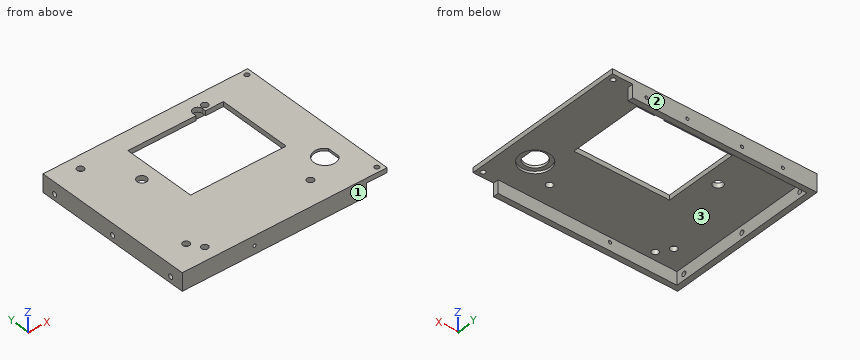
from build123d import *

# Parameters (mm, degrees)
COPYSKETCH010_W   = 150
COPYSKETCH010_H   = 120
COPYSKETCH010_R   = 2.5
COPYSKETCH010_R_2 = 3.5
COPYSKETCH010_R_3 = 1.75
PAD_DEPTH         = 3.5
PAD001_DEPTH      = 13
SKETCH001_R       = 1.75
POCKET_DEPTH      = 5
SKETCH002_R       = 1.15
POCKET001_DEPTH   = 5
SKETCH003_R       = 1.15
POCKET002_DEPTH   = 5
SKETCH004_R       = 11
POCKET003_DEPTH   = 1.75


with BuildPart() as part:
    # CopySketch010 → Pad (new body)
    with BuildSketch(Plane(origin=(0, 0, 0), x_dir=(-1, 0, 0), z_dir=(0, 0, -1))):
        with Locations((-75, 0)):
            Rectangle(COPYSKETCH010_W, COPYSKETCH010_H)
        with Locations((-110, 50)):
            Circle(COPYSKETCH010_R, mode=Mode.SUBTRACT)
        with Locations((-110, -41)):
            Circle(COPYSKETCH010_R, mode=Mode.SUBTRACT)
        with Locations((-19, -41)):
            Circle(COPYSKETCH010_R, mode=Mode.SUBTRACT)
        with Locations((-19, 50)):
            Circle(COPYSKETCH010_R, mode=Mode.SUBTRACT)
        with Locations((-38.79, 20.377)):
            Circle(COPYSKETCH010_R_2, mode=Mode.SUBTRACT)
        with Locations((-146, 56)):
            Circle(COPYSKETCH010_R_3, mode=Mode.SUBTRACT)
        with Locations((-146, -56)):
            Circle(COPYSKETCH010_R_3, mode=Mode.SUBTRACT)
        with Locations((-25, -50)):
            Circle(COPYSKETCH010_R, mode=Mode.SUBTRACT)
        with BuildLine():
            Line((-50, -8.35), (-120, -8.35))
            Line((-120, -8.35), (-120, 45.65))
            Line((-120, 45.65), (-106.908, 45.65))
            Line((-106.908, 48.264), (-106.908, 45.65))
            ThreePointArc((-99.908002, 48.26), (-103.406, 51.763999), (-106.908, 48.264))
            Line((-99.908002, 48.26), (-99.908002, 45.65))
            Line((-99.908002, 45.65), (-50, 45.65))
            Line((-50, 45.65), (-50, -8.35))
        make_face(mode=Mode.SUBTRACT)
        with BuildLine():
            ThreePointArc((-136.5, -34.66369), (-122, -30), (-136.5, -25.33631))
            Line((-136.5, -34.66369), (-136.5, -25.33631))
        make_face(mode=Mode.SUBTRACT)
    extrude(amount=PAD_DEPTH)

    # Sketch (on Face23 of Pad) → Pad001 (join)
    with BuildSketch(Plane.XY):
        Polygon((135, 60), (135, 56), (4, 56), (4, -56), (135, -56), (135, -60), (0, -60), (0, 60), align=None)
    extrude(amount=-PAD001_DEPTH)

    # Sketch001 → Pocket (cut)
    with BuildSketch(Plane.YZ):
        with Locations((0, -8.5)):
            Circle(SKETCH001_R)
        with Locations((50, -8.5)):
            Circle(SKETCH001_R)
        with Locations((-50, -8.5)):
            Circle(SKETCH001_R)
    extrude(amount=POCKET_DEPTH, mode=Mode.SUBTRACT)

    # Sketch002 → Pocket001 (cut)
    with BuildSketch(Plane.XZ.offset(60)):
        with Locations((53, -7)):
            Circle(SKETCH002_R)
    extrude(amount=-POCKET001_DEPTH, mode=Mode.SUBTRACT)

    # Sketch003 → Pocket002 (cut)
    with BuildSketch(Plane.XZ.offset(-60)):
        with Locations((25, -8)):
            Circle(SKETCH003_R)
        with Locations((125, -8)):
            Circle(SKETCH003_R)
        with Locations((95, -8)):
            Circle(SKETCH003_R)
        with Locations((55, -8)):
            Circle(SKETCH003_R)
    extrude(amount=POCKET002_DEPTH, mode=Mode.SUBTRACT)

    # Sketch004 → Pocket003 (cut)
    with BuildSketch(Plane.XY.offset(-3.5)):
        with Locations((130, -30)):
            Circle(SKETCH004_R)
    extrude(amount=POCKET003_DEPTH, mode=Mode.SUBTRACT)


solid = part.part
Geometry check sheet. Reference: the model listing, model coordinates, mm. Face numbers are marked on the shaded views. Round coordinates to 2 decimals unless told otherwise and drop trailing zeros. Order: outer loops, then holes, each group sorted by start corner. A loop starts at its lowest first (then second) coordinate and runs counter-clockwise, first axis right, second up. Notation, with made-up numbers: (-10, 29) - (43, 29) arc R18 cw to (43, 54) - close; hole circle Ø4 at (3, 77.25). An arc over 180 degrees is marked (long way). One line per question, with ' | ' between items. Start each with the question number.
(1) Sectioned sample at D-D on x = 128.5. Record the cut outline in (y, z).
(2) Sectioned sample at B-B on y = 28.5. Record the cut outline in (x, z).
(3) Sectioned sample at A-A on x = 38.79. Record the cut outline in (y, z).
(4) Thickness scan on L1, parallel to Y at x = 0.9, z = -8.5; L2, parallel to Y at x = 19, z = -0.95; L3, parallel to X at y = 57.85, z = -8. Record the ranges inside material, lowest first. Write a range as [from, to].
(5) Release check for a two-part mould opening along Y. For the marked faces 1, 2 and 3 record: released by +Y, released by -Y, zero draft, split by the parting line, or undercut.
(6) Depth check by flat-ended pin: pin 1 Ø1.8 at (x, z) = (53, -7) entering from -Y; pin 2 Ø9 at (x, y) = (38.79, 20.377) entering from -Z; pin 3 Ø11 at (x, y) = (129.5, -27) entering from -Z. Enter the tip coordinate at first touch or a pass-through.
(7) Sectioned sample at C-C on x = 110. Record the cut outline in (y, z), and give its area (3 significant figures).
Conclusion:
1) outline: (-60, -13) - (-56, -13) - (-56, -3.5) - (-40.9, -3.5) - (-40.9, -1.75) - (-37.86, -1.75) - (-37.86, 0) - (-60, 0) - close; (-22.14, -1.75) - (-19.1, -1.75) - (-19.1, -3.5) - (56, -3.5) - (56, -13) - (60, -13) - (60, 0) - (-22.14, 0) - close
2) outline: (0, -13) - (4, -13) - (4, -3.5) - (50, -3.5) - (50, 0) - (0, 0) - close; (120, -3.5) - (150, -3.5) - (150, 0) - (120, 0) - close
3) outline: (-60, -13) - (-56, -13) - (-56, -3.5) - (16.88, -3.5) - (16.88, 0) - (-60, 0) - close; (23.88, -3.5) - (56, -3.5) - (56, -13) - (60, -13) - (60, 0) - (23.88, 0) - close
4) L1: y = [-60, -51.75], [-48.25, -1.75], [1.75, 48.25], [51.75, 60] | L2: y = [-60, -43.5], [-38.5, 47.5], [52.5, 60] | L3: x = [0, 23.85], [26.15, 53.85], [56.15, 93.85], [96.15, 123.85], [126.15, 135]
5) face 1: released by -Y | face 2: released by +Y | face 3: undercut
6) pin 1: stops at y = 56 | pin 2: stops at z = -3.5 | pin 3: stops at z = -1.75
7) outline: (-60, -13) - (-56, -13) - (-56, -3.5) - (-43.5, -3.5) - (-43.5, 0) - (-60, 0) - close; (-38.5, -3.5) - (-8.35, -3.5) - (-8.35, 0) - (-38.5, 0) - close; (45.65, -3.5) - (47.5, -3.5) - (47.5, 0) - (45.65, 0) - close; (52.5, -3.5) - (56, -3.5) - (56, -13) - (60, -13) - (60, 0) - (52.5, 0) - close | area: 272 mm2
